```python
from build123d import *

# Parameters (mm, degrees)
SKETCH1_W           = 30
SKETCH1_H           = 52
BOSS_EXTRUDE1_DEPTH = 85
SKETCH2_R           = 14.25
CUT_EXTRUDE1_DEPTH  = 51
SKETCH3_R           = 11.218089099
CUT_EXTRUDE2_DEPTH  = 27
CUT_EXTRUDE3_DEPTH  = 6
CUT_EXTRUDE4_DEPTH  = 15
SKETCH4_W           = 26.454461606
SKETCH4_H           = 43.1
CUT_EXTRUDE5_DEPTH  = 28
CUT_EXTRUDE6_DEPTH  = 46
SKETCH8_W           = 25
SKETCH8_H           = 7
CUT_EXTRUDE7_DEPTH  = 8


with BuildPart() as part:
    # Sketch1 → Boss-Extrude1 (new body)
    with BuildSketch(Plane.XY):
        with Locations((-485, 30)):
            Rectangle(SKETCH1_W, SKETCH1_H)
    extrude(amount=BOSS_EXTRUDE1_DEPTH)

    # Sketch2 → Cut-Extrude1 (cut)
    with BuildSketch(Plane(origin=(0, 50, 0), x_dir=(1, 0, 0), z_dir=(0, 1, 0))):
        with Locations((-475.99810076, -62.3)):
            Circle(SKETCH2_R)
    extrude(amount=-CUT_EXTRUDE1_DEPTH, mode=Mode.SUBTRACT)

    # Sketch3 → Cut-Extrude2 (cut)
    with BuildSketch(Plane.XZ.offset(-4)):
        with Locations((-483.99810076, 62.3)):
            Circle(SKETCH3_R)
    extrude(amount=-CUT_EXTRUDE2_DEPTH, mode=Mode.SUBTRACT)

    # Sketch5 → Cut-Extrude3 (cut)
    with BuildSketch(Plane(origin=(0, 56, 0), x_dir=(1, 0, 0), z_dir=(0, 1, 0))):
        Polygon((-488.026219091, -30.701179091), (-480.468321914, -30.986702473), (-476.442102823, -24.584133211), (-479.973780909, -17.896040565), (-487.531678086, -17.610517183), (-491.557897177, -24.013086446), align=None)
    extrude(amount=-CUT_EXTRUDE3_DEPTH, mode=Mode.SUBTRACT)

    # Sketch6 → Cut-Extrude4 (cut)
    with BuildSketch(Plane(origin=(0, 56, 0), x_dir=(1, 0, 0), z_dir=(0, 1, 0))):
        with BuildLine():
            Line((-472.49810076, -79.8), (-472.49810076, -74.8))
            Line((-472.49810076, -74.8), (-479.49810076, -74.8))
            Line((-479.49810076, -74.8), (-479.49810076, -79.8))
            ThreePointArc((-479.49810076, -79.8), (-475.99810076, -83.3), (-472.49810076, -79.8))
        make_face()
        with BuildLine():
            Line((-472.49810076, -44.8), (-472.49810076, -49.8))
            Line((-472.49810076, -49.8), (-479.49810076, -49.8))
            Line((-479.49810076, -49.8), (-479.49810076, -44.8))
            ThreePointArc((-479.49810076, -44.8), (-475.99810076, -41.3), (-472.49810076, -44.8))
        make_face()
    extrude(amount=-CUT_EXTRUDE4_DEPTH, mode=Mode.SUBTRACT)

    # Sketch4 → Cut-Extrude5 (cut)
    with BuildSketch(Plane(origin=(0, 4, 0), x_dir=(-1, 0, 0), z_dir=(0, -1, 0))):
        with Locations((483.227230803, -62.15)):
            Rectangle(SKETCH4_W, SKETCH4_H)
    extrude(amount=-CUT_EXTRUDE5_DEPTH, mode=Mode.SUBTRACT)

    # Sketch7 → Cut-Extrude6 (cut)
    with BuildSketch(Plane(origin=(0, 42, 0), x_dir=(1, 0, 0), z_dir=(0, 1, 0))):
        with BuildLine():
            Line((-484, -10.298609828), (-469.568981223, -10.298609828))
            Line((-469.568981223, -10.298609828), (-469.568981223, -38.298609828))
            Line((-469.568981223, -38.298609828), (-484, -38.298609828))
            ThreePointArc((-484, -38.298609828), (-498, -24.298609828), (-484, -10.298609828))
        make_face()
    extrude(amount=-CUT_EXTRUDE6_DEPTH, mode=Mode.SUBTRACT)

    # Sketch8 → Cut-Extrude7 (cut)
    with BuildSketch(Plane(origin=(0, 0, 0), x_dir=(-1, 0, 0), z_dir=(0, 0, -1))):
        with Locations((482.5, 7.5)):
            Rectangle(SKETCH8_W, SKETCH8_H)
    extrude(amount=-CUT_EXTRUDE7_DEPTH, mode=Mode.SUBTRACT)


solid = part.part
```
Build history of the part. All positions in model axes, mm. A direction names the side the tool comes from. Coordinates: 2 decimals unless noted, no trailing zeros. Order: outer loops, then holes, each group sorted by start corner. A loop starts at its lowest first (then second) coordinate and runs counter-clockwise, first axis right, second up. Notation, with made-up numbers: (4.25, 26) -> (12.25, 26) arc R20 ccw to (12.25, 55) -> close; hole circle Ø8 at (73, 0.25). An arc over 180 degrees is marked (long way). Answer in a Markdown table with one row per item. Add a question column.
Q1. Band-saw the part on A-A, the plane y = 9.5. List the corners of the cut face in (x, z).
Q2. Band-saw the part on D-D, the plane y = 28. List the corners of the cut face in (x, z), then the cut area to 3 significant figures.
Q3. Which spindle directions (+Z, -Z, +X, -X, +Y, -Y) get a long thin tool onto all of the face, cutting with end or side? Do faces 1 (the face through (-472.498, 49, 47)), 2 (the face through (-476, 53, 49.8)), 3 (the face through (-482, 8, 8)), 4 (the face through (-484, 42, 24)). Say none if no direction does.
Q4. Wall check: line 1 along Z through (x, y) = (-471.5, 24); line 2 along Z through (x, y) = (-487, 7); line 3 along Y through (x, z) = (-474.25, 66). Give the ranges that are in metal, low to high. Write a range as [from, to].
Q5. Band-saw the part on B-B, the plane z = 62.3. List the corners of the cut face in (x, y), then the cut area to 3 significant figures.
Q6. Drop flat-ended pins along their axis: pin 1 (5.5 mm diameter, centred on x = -477, y = 8.5, fed in from -Z); pin 2 (8 mm diameter, centred on x = -485.5, z = 51.5, fed in from -Y); pin 3 (9 mm diameter, centred on x = -485, z = 2.5, fed in from -Y); pin 4 (12 mm diameter, centred on y = 36, z = 69, fed in from +X). Give the stop position or say it passes through.
Q7. Band-saw the part on C-C, the plane x = -481.5. List the corners of the cut face in (y, z), then the cut area to 3 significant figures.
Q8. Mould opens along X. For faces 5 (the face through (-476, 53, 74.8)), 6 (the face through (-476.1, 48.6, 83.3)), 7 (the face through (-495, 7, 4)), 8 (the face through (-485, 30, 0)) say: +X half, -X half, draft (parallel to the pull), parting line (faces both ways), or undercut.
Answers follow:
| question | item | result |
|---|---|---|
| 1 | outline | (-500, 0) -> (-495, 0) -> (-495, 8) -> (-470, 8) -> (-470, 10.3) -> (-484, 10.3) arc R14 cw to (-484, 38.3) -> (-470, 38.3) -> (-470, 40.6) -> (-496.45, 40.6) -> (-496.45, 83.7) -> (-470, 83.7) -> (-470, 85) -> (-500, 85) -> close |
| 2 | outline | (-500, 0) -> (-470, 0) -> (-470, 10.3) -> (-484, 10.3) arc R14 cw to (-484, 38.3) -> (-470, 38.3) -> (-470, 40.6) -> (-496.45, 40.6) -> (-496.45, 83.7) -> (-470, 83.7) -> (-470, 85) -> (-500, 85) -> close |
| 2 | area | 710 mm^2 |
| 3 | face 1 | +Y |
| 3 | face 2 | +Y, -Y |
| 3 | face 3 | -Z, +X, -Y |
| 3 | face 4 | +X, -Y |
| 4 | line 1 | [0, 10.3], [38.3, 40.6], [83.7, 85] |
| 4 | line 2 | [8, 10.62], [37.97, 40.6], [83.7, 85] |
| 4 | line 3 | [50, 56] |
| 5 | outline | (-500, 4) -> (-496.45, 4) -> (-496.45, 32) -> (-490.25, 32) -> (-490.25, 50) -> (-470, 50) -> (-470, 56) -> (-500, 56) -> close |
| 5 | area | 455 mm^2 |
| 6 | pin 1 | z = 0 |
| 6 | pin 2 | y = 32 |
| 6 | pin 3 | y = 11 |
| 6 | pin 4 | x = -482.46 |
| 7 | outline | (4, 8) -> (11, 8) -> (11, 0) -> (56, 0) -> (56, 17.84) -> (50, 17.84) -> (50, 30.95) -> (56, 30.95) -> (56, 85) -> (4, 85) -> (4, 83.7) -> (32, 83.7) -> (32, 75.45) -> (50, 75.45) -> (50, 49.15) -> (32, 49.15) -> (32, 40.6) -> (4, 40.6) -> (4, 38.3) -> (42, 38.3) -> (42, 10.3) -> (4, 10.3) -> close |
| 7 | area | 1,540 mm^2 |
| 8 | face 5 | undercut |
| 8 | face 6 | undercut |
| 8 | face 7 | +X half |
| 8 | face 8 | draft |
